The model under review builds one solid part; all positions refer to its coordinate system, in mm. A direction names the side the tool comes from. Give positions to 0.01 mm unless a question says otherwise; leave off trailing zeros. Order: outer loops, then holes, each group sorted by start corner. A loop starts at its lowest first (then second) coordinate and runs counter-clockwise, first axis right, second up. Notation, with made-up numbers: (3.5, 37) -> (12.5, 37) arc R18 cw to (12.5, 47) -> close; hole circle Ø8 at (19, 77.5). An arc over 180 degrees is marked (long way). Use one line per item in the form item = value.
```python
from build123d import *

# Parameters (mm, degrees)
BOSS_EXTRUDE1_DEPTH = 5
FILLET1_R           = 20


with BuildPart() as part:
    # Sketch1 → Boss-Extrude1 (new, symmetric)
    with BuildSketch(Plane(origin=(0, 0, 0), x_dir=(1, 0, 0), z_dir=(0, 1, 0))):
        with BuildLine():
            Line((-13.413143077, 1.086856923), (-14.5, 0))
            ThreePointArc((-14.5, 0), (-14.497902835, -0.246603683), (-14.491611948, -0.493136032))
            Line((-14.491611948, -0.493136032), (-13.398098019, -1.258822728))
            Line((-13.398098019, -1.258822728), (-14.279712419, -2.517898576))
            ThreePointArc((-14.279712419, -2.517898576), (-14.234824835, -2.760391626), (-14.185819627, -3.002086193))
            Line((-14.185819627, -3.002086193), (-12.975958532, -3.566253687))
            Line((-12.975958532, -3.566253687), (-13.625543001, -4.959292078))
            ThreePointArc((-13.625543001, -4.959292078), (-13.539228884, -5.190306466), (-13.448998355, -5.419819485))
            Line((-13.448998355, -5.419819485), (-12.159551111, -5.765325833))
            Line((-12.159551111, -5.765325833), (-12.557368355, -7.25))
            ThreePointArc((-12.557368355, -7.25), (-12.432250316, -7.462516471), (-12.303536073, -7.672874305))
            Line((-12.303536073, -7.672874305), (-10.973681883, -7.789221471))
            Line((-10.973681883, -7.789221471), (-11.107644425, -9.32042034))
            ThreePointArc((-11.107644425, -9.32042034), (-10.947524112, -9.50798169), (-10.784237074, -9.692792721))
            Line((-10.784237074, -9.692792721), (-9.454382883, -9.576445555))
            Line((-9.454382883, -9.576445555), (-9.32042034, -11.107644425))
            ThreePointArc((-9.32042034, -11.107644425), (-9.130162928, -11.264551696), (-8.937264488, -11.418200536))
            Line((-8.937264488, -11.418200536), (-7.647817244, -11.072694188))
            Line((-7.647817244, -11.072694188), (-7.25, -12.557368355))
            ThreePointArc((-7.25, -12.557368355), (-7.035386364, -12.678853998), (-6.818737643, -12.796672105))
            Line((-6.818737643, -12.796672105), (-5.608876548, -12.232504611))
            Line((-5.608876548, -12.232504611), (-4.959292078, -13.625543001))
            ThreePointArc((-4.959292078, -13.625543001), (-4.726843145, -13.707915738), (-4.493026906, -13.786323267))
            Line((-4.493026906, -13.786323267), (-3.399512976, -13.020636571))
            Line((-3.399512976, -13.020636571), (-2.517898576, -14.279712419))
            ThreePointArc((-2.517898576, -14.279712419), (-2.274677189, -14.320469395), (-2.030797819, -14.357083973))
            Line((-2.030797819, -14.357083973), (-1.086856923, -13.413143077))
            Line((-1.086856923, -13.413143077), (0, -14.5))
            ThreePointArc((0, -14.5), (0.246603683, -14.497902835), (0.493136032, -14.491611948))
            Line((0.493136032, -14.491611948), (1.258822728, -13.398098019))
            Line((1.258822728, -13.398098019), (2.517898576, -14.279712419))
            ThreePointArc((2.517898576, -14.279712419), (2.760391626, -14.234824835), (3.002086193, -14.185819627))
            Line((3.002086193, -14.185819627), (3.566253687, -12.975958532))
            Line((3.566253687, -12.975958532), (4.959292078, -13.625543001))
            ThreePointArc((4.959292078, -13.625543001), (5.190306466, -13.539228884), (5.419819485, -13.448998355))
            Line((5.419819485, -13.448998355), (5.765325833, -12.159551111))
            Line((5.765325833, -12.159551111), (7.25, -12.557368355))
            ThreePointArc((7.25, -12.557368355), (7.462516471, -12.432250316), (7.672874305, -12.303536073))
            Line((7.672874305, -12.303536073), (7.789221471, -10.973681883))
            Line((7.789221471, -10.973681883), (9.32042034, -11.107644425))
            ThreePointArc((9.32042034, -11.107644425), (9.50798169, -10.947524112), (9.692792721, -10.784237074))
            Line((9.692792721, -10.784237074), (9.576445555, -9.454382883))
            Line((9.576445555, -9.454382883), (11.107644425, -9.32042034))
            ThreePointArc((11.107644425, -9.32042034), (11.264551696, -9.130162928), (11.418200536, -8.937264488))
            Line((11.418200536, -8.937264488), (11.072694188, -7.647817244))
            Line((11.072694188, -7.647817244), (12.557368355, -7.25))
            ThreePointArc((12.557368355, -7.25), (12.678853998, -7.035386364), (12.796672105, -6.818737643))
            Line((12.796672105, -6.818737643), (12.232504611, -5.608876548))
            Line((12.232504611, -5.608876548), (13.625543001, -4.959292078))
            ThreePointArc((13.625543001, -4.959292078), (13.707915738, -4.726843145), (13.786323267, -4.493026906))
            Line((13.786323267, -4.493026906), (13.020636571, -3.399512976))
            Line((13.020636571, -3.399512976), (14.279712419, -2.517898576))
            ThreePointArc((14.279712419, -2.517898576), (14.320469395, -2.274677189), (14.357083973, -2.030797819))
            Line((14.357083973, -2.030797819), (13.413143077, -1.086856923))
            Line((13.413143077, -1.086856923), (14.5, 0))
            ThreePointArc((14.5, 0), (14.497902835, 0.246603683), (14.491611948, 0.493136032))
            Line((14.491611948, 0.493136032), (13.398098019, 1.258822728))
            Line((13.398098019, 1.258822728), (14.279712419, 2.517898576))
            ThreePointArc((14.279712419, 2.517898576), (14.234824835, 2.760391626), (14.185819627, 3.002086193))
            Line((14.185819627, 3.002086193), (12.975958532, 3.566253687))
            Line((12.975958532, 3.566253687), (13.625543001, 4.959292078))
            ThreePointArc((13.625543001, 4.959292078), (13.539228884, 5.190306466), (13.448998355, 5.419819485))
            Line((13.448998355, 5.419819485), (12.159551111, 5.765325833))
            Line((12.159551111, 5.765325833), (12.557368355, 7.25))
            ThreePointArc((12.557368355, 7.25), (12.432250316, 7.462516471), (12.303536073, 7.672874305))
            Line((12.303536073, 7.672874305), (10.973681883, 7.789221471))
            Line((10.973681883, 7.789221471), (11.107644425, 9.32042034))
            ThreePointArc((11.107644425, 9.32042034), (10.947524112, 9.50798169), (10.784237074, 9.692792721))
            Line((10.784237074, 9.692792721), (9.454382883, 9.576445555))
            Line((9.454382883, 9.576445555), (9.32042034, 11.107644425))
            ThreePointArc((9.32042034, 11.107644425), (9.130162928, 11.264551696), (8.937264488, 11.418200536))
            Line((8.937264488, 11.418200536), (7.647817244, 11.072694188))
            Line((7.647817244, 11.072694188), (7.25, 12.557368355))
            ThreePointArc((7.25, 12.557368355), (7.035386364, 12.678853998), (6.818737643, 12.796672105))
            Line((6.818737643, 12.796672105), (5.608876548, 12.232504611))
            Line((5.608876548, 12.232504611), (4.959292078, 13.625543001))
            ThreePointArc((4.959292078, 13.625543001), (4.726843145, 13.707915738), (4.493026906, 13.786323267))
            Line((4.493026906, 13.786323267), (3.399512976, 13.020636571))
            Line((3.399512976, 13.020636571), (2.517898576, 14.279712419))
            ThreePointArc((2.517898576, 14.279712419), (2.274677189, 14.320469395), (2.030797819, 14.357083973))
            Line((2.030797819, 14.357083973), (1.086856923, 13.413143077))
            Line((1.086856923, 13.413143077), (0, 14.5))
            ThreePointArc((0, 14.5), (-0.246603683, 14.497902835), (-0.493136032, 14.491611948))
            Line((-0.493136032, 14.491611948), (-1.258822728, 13.398098019))
            Line((-1.258822728, 13.398098019), (-2.517898576, 14.279712419))
            ThreePointArc((-2.517898576, 14.279712419), (-2.760391626, 14.234824835), (-3.002086193, 14.185819627))
            Line((-3.002086193, 14.185819627), (-3.566253687, 12.975958532))
            Line((-3.566253687, 12.975958532), (-4.959292078, 13.625543001))
            ThreePointArc((-4.959292078, 13.625543001), (-5.190306466, 13.539228884), (-5.419819485, 13.448998355))
            Line((-5.419819485, 13.448998355), (-5.765325833, 12.159551111))
            Line((-5.765325833, 12.159551111), (-7.25, 12.557368355))
            ThreePointArc((-7.25, 12.557368355), (-7.462516471, 12.432250316), (-7.672874305, 12.303536073))
            Line((-7.672874305, 12.303536073), (-7.789221471, 10.973681883))
            Line((-7.789221471, 10.973681883), (-9.32042034, 11.107644425))
            ThreePointArc((-9.32042034, 11.107644425), (-9.50798169, 10.947524112), (-9.692792721, 10.784237074))
            Line((-9.692792721, 10.784237074), (-9.576445555, 9.454382883))
            Line((-9.576445555, 9.454382883), (-11.107644425, 9.32042034))
            ThreePointArc((-11.107644425, 9.32042034), (-11.264551696, 9.130162928), (-11.418200536, 8.937264488))
            Line((-11.418200536, 8.937264488), (-11.072694188, 7.647817244))
            Line((-11.072694188, 7.647817244), (-12.557368355, 7.25))
            ThreePointArc((-12.557368355, 7.25), (-12.678853998, 7.035386364), (-12.796672105, 6.818737643))
            Line((-12.796672105, 6.818737643), (-12.232504611, 5.608876548))
            Line((-12.232504611, 5.608876548), (-13.625543001, 4.959292078))
            ThreePointArc((-13.625543001, 4.959292078), (-13.707915738, 4.726843145), (-13.786323267, 4.493026906))
            Line((-13.786323267, 4.493026906), (-13.020636571, 3.399512976))
            Line((-13.020636571, 3.399512976), (-14.279712419, 2.517898576))
            ThreePointArc((-14.279712419, 2.517898576), (-14.320469395, 2.274677189), (-14.357083973, 2.030797819))
            Line((-14.357083973, 2.030797819), (-13.413143077, 1.086856923))
        make_face()
    extrude(amount=BOSS_EXTRUDE1_DEPTH, both=True)

    # Sketch2 → Revolve1 (revolve)
    with BuildSketch(Plane(origin=(0, 0, 0), x_dir=(0, 0, -1), z_dir=(1, 0, 0)), mode=Mode.PRIVATE) as revolve1_sk:
        with BuildLine():
            Line((22.10493006, 19.026987327), (25.061867778, 19.026987327))
            Line((25.061867778, 19.026987327), (25.061867778, 105.264393418))
            Line((25.061867778, 105.264393418), (0, 105.264393418))
            Line((0, 105.264393418), (0, 0))
            Line((0, 0), (12.10493006, 0))
            Line((12.10493006, 0), (12.10493006, 9.026987327))
            ThreePointArc((12.10493006, 9.026987327), (15.033862249, 16.098055139), (22.10493006, 19.026987327))
        make_face()
    revolve(revolve1_sk.sketch.rotate(Axis((0, 105.264393418, 0), (0, -1, 0)), 180), axis=Axis((0, 105.264393418, 0), (0, -1, 0)))

    # Fillet1
    fillet1_edges = [part.edges().sort_by_distance(p)[0] for p in [
        (0, 19.026987327, -25.061867778),
    ]]
    fillet(fillet1_edges, radius=FILLET1_R)


solid = part.part
```
1. Add section A-A on y = 52.5. Give the boundary of the cut face in (x, z).
Values:
outline = circle Ø50.12 at (0, 0)
2. For pin 1 Ø4 at (y, z) = (21, 16.5) entering from +X; pin 2 Ø3 at (y, z) = (41, -3) entering from -X; pin 3 Ø1.5 at (x, y) = (-7, 55) entering from -Z, all flat-tipped, find the tip position at first contact; note any pin that passes through.
Values:
pin_1 = 15.41
pin_2 = -25.02
pin_3 = -24.27
3. For L1, parallel to Y at x = 5.5, z = 12; L2, parallel to X at y = 2, z = 0; L3, parallel to Z at x = -3, y = 98, list the stretches that pass through material, from the lowest coordinate up.
Values:
L1 = -5 to 5, 13.58 to 105.26
L2 = -14.5 to 14.5
L3 = -24.88 to 24.88
4. The part is to be moulded in two halves that separate along Y. For faces 1 (the face through (0, -5, 0)), 2 (the face through (0, 105.264, 0)), 3 (the face through (3, 5, 12)), say which applies: +Y half, -Y half, draft (parallel to the pull), parting line (faces both ways), or undercut.
Values:
face_1 = -Y half
face_2 = +Y half
face_3 = undercut
5. Tool access review of faces 4 (the face through (-3.636, 7.042, 11.546)), 5 (the face through (-24.85, 69.99, -3.26)): name each direction out of +Z, -Z, +X, -X, +Y, -Y from which nothing blocks a thin tool from reaching the whole face with its end or side.
Values:
face_4 = none
face_5 = +Y, -Y
